Verification items for this drawing (mm, ordinates from the low corner). A direction names the side the tool comes from. Coordinates: 2 decimals unless noted, no trailing zeros. Order: outer loops, then holes, each group sorted by start corner. A loop starts at its lowest first (then second) coordinate and runs counter-clockwise, first axis right, second up. Notation, with made-up numbers: M -22.75,23 L -9.75,23 A28 ccw -9.75,58 Z; hole C -21,25.25 d10. An arc over 180 degrees is marked long. Return JSON: item names as keys, results as strings. Group by question number.
1. Material ranges on line 1 along Z through (x, y) = (3, 7.5); line 2 along X through (y, z) = (4.75, 6); line 3 along X through (y, z) = (5.5, 7), recorded low to high.
2. Section check A-A, the plane z = 3.5. Record the cut outline in (x, y), plus the area to 3 significant figures.
3. Section check C-C, the plane z = 1.5. Record the cut outline in (x, y), plus the area to 3 significant figures.
4. Section check B-B, the plane x = 1. Record the cut outline in (y, z).
5. Section check D-D, the plane x = 7.5. Record the cut outline in (y, z), plus the area to 3 significant figures.
6. Gauge pin test, flat ends, axial feed: pin 1 (2 mm diameter, centred on x = 2.5, z = 10, fed in from +Y); pin 2 (2 mm diameter, centred on x = 6, y = 5.5, fed in from +Z); pin 3 (4 mm diameter, centred on y = 5.5, z = 7.5, fed in from +X). Record the tip position at first contact, or that the pin passes through.
7. Set-up check for the marked faces 1 and 2: record each of +Z, -Z, +X, -X, +Y, -Y from which the full face is reachable in a straight line by a thin tool's end or side.
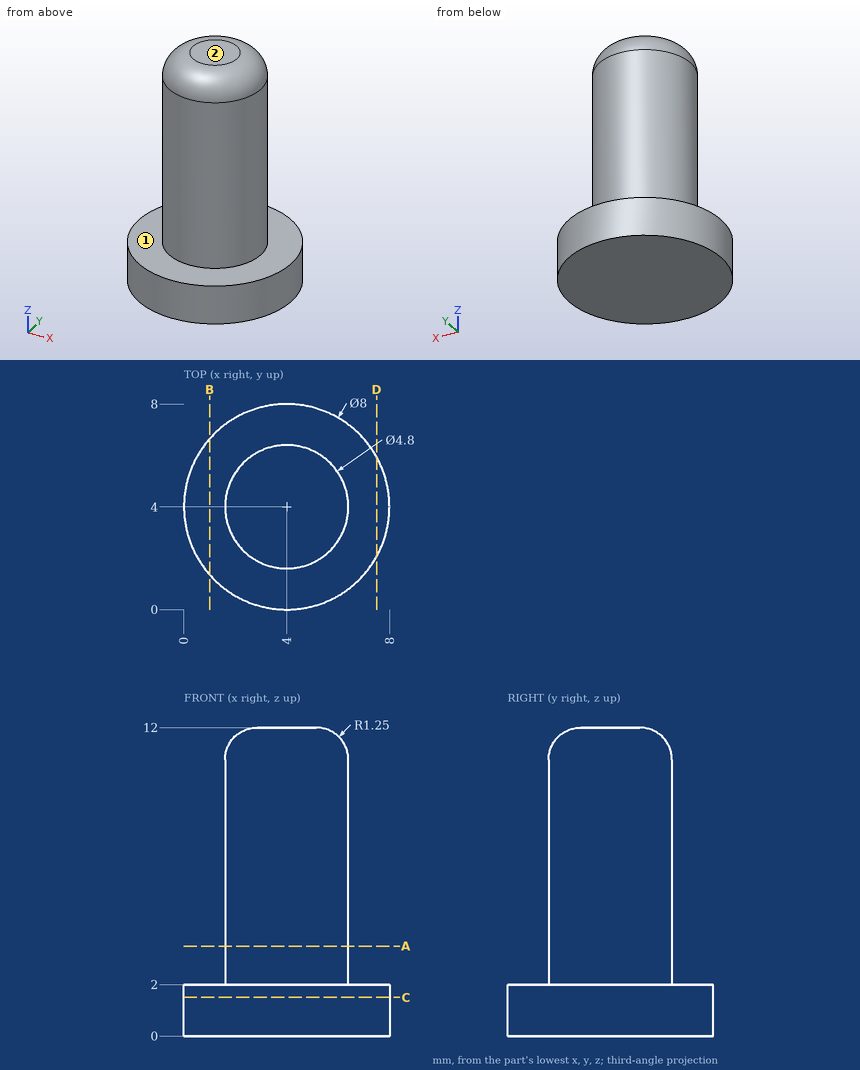
Answers follow:
{
 "1": {"line 1": "0 to 2", "line 2": "1.72 to 6.28", "line 3": "2.13 to 5.87"},
 "2": {"outline": "C 4,4 d4.8", "area": "18.1 mm^2"},
 "3": {"outline": "C 4,4 d8", "area": "50.3 mm^2"},
 "4": {"outline": "M 1.35,0 L 6.65,0 L 6.65,2 L 1.35,2 Z"},
 "5": {"outline": "M 2.06,0 L 5.94,0 L 5.94,2 L 2.06,2 Z", "area": "7.75 mm^2"},
 "6": {"pin 1": "y = 6.35", "pin 2": "z = 11.95", "pin 3": "x = 6.4"},
 "7": {"face 1": "+Z", "face 2": "+Z, +X, -X, +Y, -Y"}
}
